For this review, take the finished solid that the model builds, in its own axes (mm). Face numbers are marked on the shaded views. A direction names the side the tool comes from. Coordinates: 2 decimals unless noted, no trailing zeros. Loops run counter-clockwise (first coordinate to the right, second up) from the corner with the lowest first, then second, coordinate; pieces in that order, holes last. Notation, with made-up numbers: (17.5, 59.25) - (21.5, 59.25) arc R30 cw to (21.5, 83.25) - close; hole circle Ø6 at (36.5, -27.5). An arc over 180 degrees is marked (long way). Answer as a JSON object with one key per item and string values. Group by question number.
Item 1: We need section C-C (x = 0). Give the boundary of the cut face in (y, z), then the cut area to 3 significant figures.
Item 2: Clearance check with flat-ended pins moving along their axes: pin 1 (1.5 mm diameter, centred on x = 1.5, y = 25.5, fed in from -Z); pin 2 (10 mm diameter, centred on x = 7, y = 4.5, fed in from +Z); pin 3 (4.5 mm diameter, centred on x = 1.5, z = 0.5, fed in from -Y); pin 4 (3 mm diameter, centred on x = 0, z = 0, fed in from -Y). State where each tip first meets the part, or that it passes through.
Item 3: To check wall thickness, follow line 1 (X direction, y = 22.75, z = 0); line 2 (Y direction, x = -2, z = -2). State the ranges of each line that lie inside material, in increasing order.
Item 4: We need section B-B (y = 14.5). Give the boundary of the cut face in (x, z).
Item 5: Mouldability with a two-part tool opening along Z and no side actions: class the marked faces 1, 2 and 3 as released by +Z, released by -Z, zero draft, split by the parting line, or undercut.
Item 6: We need section A-A (z = 0). Give the boundary of the cut face in (x, y), then the cut area to 3 significant figures.
Item 7: Tool access review of the marked faces 4, 5 and 6: name each direction out of +Z, -Z, +X, -X, +Y, -Y from which nothing blocks a thin tool from reaching the whole face with its end or side.
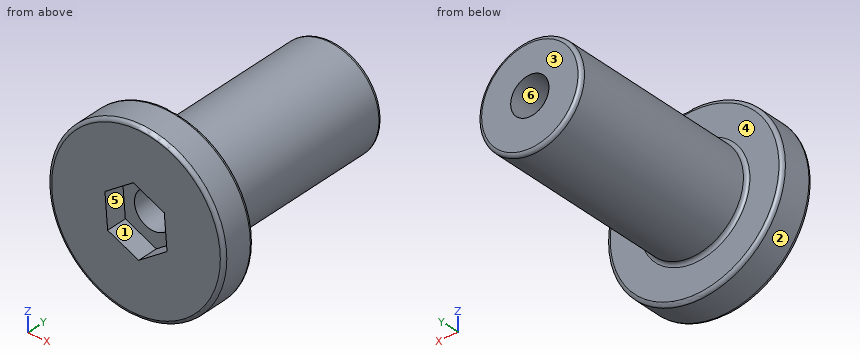
from build123d import *

# Parameters (mm, degrees)
SKETCH1_R           = 12.4
BOSS_EXTRUDE1_DEPTH = 5
SKETCH2_R           = 7.3
BOSS_EXTRUDE2_DEPTH = 28
SKETCH3_R           = 2.7
CUT_EXTRUDE1_DEPTH  = 34
CUT_EXTRUDE2_DEPTH  = 3
FILLET1_R           = 0.5


with BuildPart() as part:
    # Sketch1 → Boss-Extrude1 (new body)
    with BuildSketch(Plane(origin=(0, 0, 0), x_dir=(1, 0, 0), z_dir=(0, 1, 0))):
        Circle(SKETCH1_R)
    extrude(amount=BOSS_EXTRUDE1_DEPTH)

    # Sketch2 → Boss-Extrude2 (add)
    with BuildSketch(Plane(origin=(0, 5, 0), x_dir=(1, 0, 0), z_dir=(0, 1, 0))):
        Circle(SKETCH2_R)
    extrude(amount=BOSS_EXTRUDE2_DEPTH)

    # Sketch3 → Cut-Extrude1 (cut, through all)
    with BuildSketch(Plane(origin=(0, 33, 0), x_dir=(1, 0, 0), z_dir=(0, 1, 0))):
        Circle(SKETCH3_R)
    extrude(amount=-CUT_EXTRUDE1_DEPTH, mode=Mode.SUBTRACT)

    # Sketch4 → Cut-Extrude2 (cut)
    with BuildSketch(Plane.XZ):
        Polygon((-4.38019792, 2.081793981), (-3.992985433, -2.752465682), (0.387212487, -4.834259663), (4.38019792, -2.081793981), (3.992985433, 2.752465682), (-0.387212487, 4.834259663), align=None)
    extrude(amount=-CUT_EXTRUDE2_DEPTH, mode=Mode.SUBTRACT)

    # Fillet1
    fillet1_edges = [part.edges().sort_by_distance(p)[0] for p in [
        (-12.4, 0, 0),
        (-12.4, 5, 0),
        (-7.3, 5, 0),
        (-7.3, 33, 0),
    ]]
    fillet(fillet1_edges, radius=FILLET1_R)


solid = part.part
Check sheet entries:
{
 "1": {"outline": "(0, -11.9) arc R0.5 ccw to (0.5, -12.4) - (4.5, -12.4) arc R0.5 ccw to (5, -11.9) - (5, -7.8) arc R0.5 cw to (5.5, -7.3) - (32.5, -7.3) arc R0.5 ccw to (33, -6.8) - (33, -2.7) - (3, -2.7) - (3, -4.65) - (0, -4.65) - close; (0, 4.65) - (3, 4.65) - (3, 2.7) - (33, 2.7) - (33, 6.8) arc R0.5 ccw to (32.5, 7.3) - (5.5, 7.3) arc R0.5 cw to (5, 7.8) - (5, 11.9) arc R0.5 ccw to (4.5, 12.4) - (0.5, 12.4) arc R0.5 ccw to (0, 11.9) - close", "area": "343 mm2"},
 "2": {"pin 1": "stops at z = -7.26", "pin 2": "stops at z = 12.24", "pin 3": "stops at y = 3", "pin 4": "passes through"},
 "3": {"line 1": "x = -7.3 to -2.7, 2.7 to 7.3", "line 2": "y = 3 to 33"},
 "4": {"outline": "circle Ø14.6 at (0, 0); hole circle Ø5.4 at (0, 0)"},
 "5": {"face 1": "undercut", "face 2": "split by the parting line", "face 3": "zero draft"},
 "6": {"outline": "(-12.4, 0.5) arc R0.5 ccw to (-11.9, 0) - (-4.21, 0) - (-4.21, 3) - (-2.7, 3) - (-2.7, 33) - (-6.8, 33) arc R0.5 ccw to (-7.3, 32.5) - (-7.3, 5.5) arc R0.5 cw to (-7.8, 5) - (-11.9, 5) arc R0.5 ccw to (-12.4, 4.5) - close; (2.7, 3) - (4.21, 3) - (4.21, 0) - (11.9, 0) arc R0.5 ccw to (12.4, 0.5) - (12.4, 4.5) arc R0.5 ccw to (11.9, 5) - (7.8, 5) arc R0.5 cw to (7.3, 5.5) - (7.3, 32.5) arc R0.5 ccw to (6.8, 33) - (2.7, 33) - close", "area": "345 mm2"},
 "7": {"face 4": "+Y", "face 5": "-Y", "face 6": "+Y, -Y"}
}
